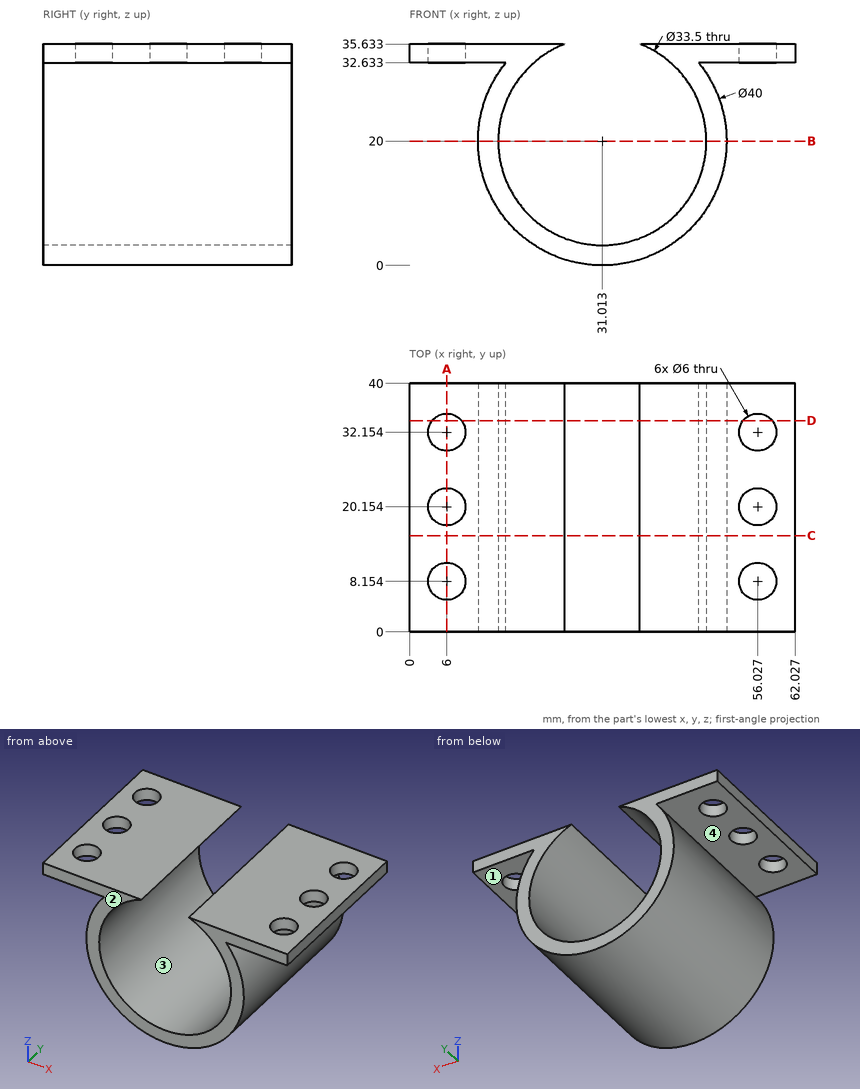
Verification items for this drawing (mm, ordinates from the low corner). A direction names the side the tool comes from. Give positions to 0.01 mm unless a question says otherwise; leave off trailing zeros. Write each loop counter-clockwise with the first axis right and the second up, starting at its lowest first coordinate (ties: lowest second). Pieces come first, ordered by that corner, then holes. Notation, with made-up numbers: (62.5, 4.25) -> (103.5, 4.25) arc R20 ccw to (103.5, 21.25) -> close; hole circle Ø7 at (48, 9). An arc over 180 degrees is marked (long way). Use CSV: the item, a comma, the result in double quotes. Start each with the question number.
Q1. Cross-section at D-D on y = 34. Count the separate pieces of the cut face and the enclosed holes in it, and give its area (3 significant figures).
Q2. Depth check by flat-ended pin: P1, Ø4, axis at y = 18.5, z = 27, coming from the +X side; P2, Ø17, axis at x = 10.5, y = 18, coming from the -Z side; P3, Ø4, axis at x = 32, y = 35.5, coming from the -Z side; P4, Ø8, axis at x = 56.03, y = 20.15, coming from the +Z side. Enter the tip coordinate at first touch or a pass-through.
Q3. Cross-section at C-C on y = 15.5. Enter the section's corners in (x, z).
Q4. Release check for a two-part mould opening along X. For the marked faces 3 and 4 record: +X half, -X half, draft (parallel to the pull), parting line (faces both ways), or undercut.
Q5. Cross-section at B-B on z = 20. Enter the section's corners in (x, y), and give its area (3 significant figures).
Q6. Tool access check on the marked faces 1 and 2. Record the directions out of +Z, -Z, +X, -X, +Y, -Y that give a thin tool (end or side, any length) a straight path to the whole face; none if there is none.
Q7. Cross-section at A-A on x = 6. Enter the section's corners in (y, z) (1 decimal).
Q8. Scan lines: line 1 along X through (y, z) = (17.5, 20); line 2 along Y through (x, z) = (6, 34.1) (1 decimal); line 3 along Z through (x, y) = (51.5, 20). Record each from-to range of solid material in increasing order.
Working result:
1,separate pieces,"3"
1,enclosed holes,"0"
1,area,"383 mm^2"
2,P1,"stops at x = 50.38"
2,P2,"stops at z = 4.01"
2,P3,"stops at z = 0"
2,P4,"stops at z = 35.63"
3,outline,"(0, 32.63) -> (15.51, 32.63) arc R20 ccw (long way) to (46.52, 32.63) -> (62.03, 32.63) -> (62.03, 35.63) -> (37.03, 35.63) arc R16.75 cw (long way) to (25, 35.63) -> (0, 35.63) -> close"
4,face 3,"undercut"
4,face 4,"draft"
5,outline,"(11.01, 0) -> (14.26, 0) -> (14.26, 40) -> (11.01, 40) -> close; (47.76, 0) -> (51.01, 0) -> (51.01, 40) -> (47.76, 40) -> close"
5,area,"260 mm^2"
6,face 1,"+X, +Y, -Y"
6,face 2,"+Z, -Z, +X, -X, -Y"
7,outline,"(0, 32.6) -> (5.2, 32.6) -> (5.2, 35.6) -> (0, 35.6) -> close; (11.2, 32.6) -> (17.2, 32.6) -> (17.2, 35.6) -> (11.2, 35.6) -> close; (23.2, 32.6) -> (29.2, 32.6) -> (29.2, 35.6) -> (23.2, 35.6) -> close; (35.2, 32.6) -> (40, 32.6) -> (40, 35.6) -> (35.2, 35.6) -> close"
8,line 1,"x = 11.01 to 14.26, 47.76 to 51.01"
8,line 2,"y = 0 to 5.2, 11.2 to 17.2, 23.2 to 29.2, 35.2 to 40"
8,line 3,"z = 32.63 to 35.63"
